from build123d import *

# Parameters (mm, degrees)
F0_R        = 1.15
F1_DEPTH    = 4
F2_R        = 1.5
F3_DEPTH    = 5
F4_T1_DEPTH = 16
F5_R        = 0.49999


# Not quite as in the source:
# - a fillet or chamfer that OpenCascade refuses, or shapes differently, is made with other operations: its cross-section is extruded or revolved along the edge and cut away or added
# - a fillet or chamfer is up to 0.001 mm smaller than in the source, because OpenCascade refuses the exact size


with BuildPart() as f1:
    # F0 (on Front) → F1 (new body)
    with BuildSketch(Plane.XZ):
        with BuildLine():
            Line((-3.5, -3.1), (5, -3.1))
            Line((5, -3.1), (5, 3.1))
            Line((5, 3.1), (-3.5, 3.1))
            ThreePointArc((-3.5, 3.1), (-3.9393398282, 2.0393398282), (-5, 1.6))
            Line((-5, 1.6), (-5, -1.6))
            ThreePointArc((-5, -1.6), (-3.9393398282, -2.0393398282), (-3.5, -3.1))
        make_face()
        with Locations((2.7, 0)):
            Circle(F0_R, mode=Mode.SUBTRACT)
    extrude(amount=F1_DEPTH)

    # F2 (on face) → F3 (cut)
    with BuildSketch(Plane(origin=(-5, 0, 0), x_dir=(0, -1, 0), z_dir=(-1, 0, 0))):
        with Locations((2, 0)):
            Circle(F2_R)
    extrude(amount=-F3_DEPTH, mode=Mode.SUBTRACT)

    # F4: fillet of radius 1.5 on 4 edges, made by hand

    # F4_s2 → F4_t1 (cut)
    with BuildSketch(Plane.YZ.offset(-7.25)):
        with BuildLine():
            ThreePointArc((0, 1.6), (-0.4393398282, 2.6606601718), (-1.5, 3.1))
            Line((-1.5, 3.1), (0, 3.1))
            Line((0, 3.1), (0, 1.6))
        make_face()
        with BuildLine():
            ThreePointArc((-4, 1.6), (-3.5606601718, 2.6606601718), (-2.5, 3.1))
            Line((-2.5, 3.1), (-4, 3.1))
            Line((-4, 3.1), (-4, 1.6))
        make_face()
        with BuildLine():
            ThreePointArc((-2.5, -3.1), (-3.5606601718, -2.6606601718), (-4, -1.6))
            Line((-4, -1.6), (-4, -3.1))
            Line((-4, -3.1), (-2.5, -3.1))
        make_face()
        with BuildLine():
            ThreePointArc((-1.5, -3.1), (-0.4393398282, -2.6606601718), (0, -1.6))
            Line((0, -1.6), (0, -3.1))
            Line((0, -3.1), (-1.5, -3.1))
        make_face()
    extrude(amount=F4_T1_DEPTH, mode=Mode.SUBTRACT)

    # F5 (radius 0.5 in the source; OpenCascade refuses exactly that, so slightly less here)
    f5_edges = [f1.edges().sort_by_distance(p)[0] for p in [
        (-5, 0, 0),
        (-5, -4, 0),
    ]]
    fillet(f5_edges, radius=F5_R)


solid = f1.part
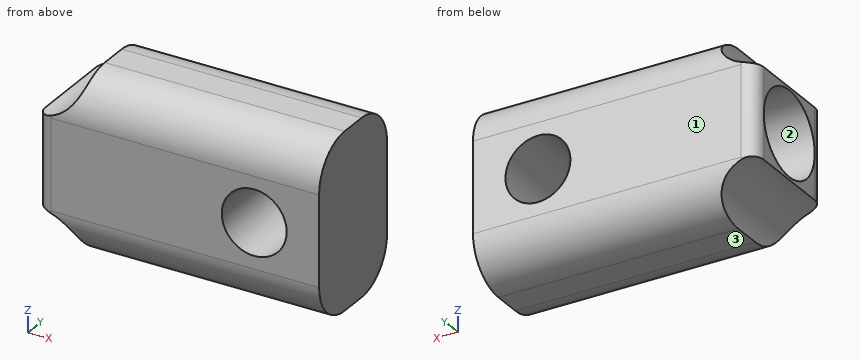
The listing builds one solid part. Answer for the finished solid, in the listing's coordinates (mm). Face numbers are marked on the shaded views. Round coordinates to 2 decimals unless told otherwise and drop trailing zeros. Order: outer loops, then holes, each group sorted by start corner. A loop starts at its lowest first (then second) coordinate and runs counter-clockwise, first axis right, second up. Notation, with made-up numbers: (65.5, 74.5) - (96.5, 74.5) arc R10 cw to (96.5, 78.5) - close; hole circle Ø6 at (38.25, 45.25). An arc over 180 degrees is marked (long way). Write item = value, one per line. Start each with the question number.
1) Given pin 1 (1.8 mm diameter, centred on x = 2.7, z = 0, fed in from +Y), flat-ended and moving along its own axis, determine where the tip first touches the part or whether it passes through.
2) Section D-D, the plane x = 0.25 is taken. Write down the section's boundary in (y, z).
3) Section B-B, the plane x = 2.7 is taken. Write down the section's boundary in (y, z), plus the area to 3 significant figures.
4) Section C-C, the plane y = -2 is taken. Write down the section's boundary in (x, z), plus the area to 3 significant figures.
5) For a pull along Y with two mould halves and no side action, classify the marked faces 1, 2 and 3 as released by +Y, released by -Y, zero draft, split by the parting line, or undercut.
6) Straight lines are drawn through the part: L1, parallel to Z at x = 2.7, y = -2; L2, parallel to X at y = -2.3, z = 0.5; L3, parallel to X at y = -2.1, z = 1. For each, find the intervals that lie inside material, in ascending order.
Results list:
q1.pin_1 = through
q2.outline = (-4, -1.6) arc R1.5 ccw to (-2.5, -3.1) - (-1.5, -3.1) arc R1.5 ccw to (0, -1.6) - (0, 1.6) arc R1.5 ccw to (-1.5, 3.1) - (-2.5, 3.1) arc R1.5 ccw to (-4, 1.6) - close
q3.outline = (-4, -1.6) arc R1.5 ccw to (-2.5, -3.1) - (-1.5, -3.1) arc R1.5 ccw to (0, -1.6) - (0, -1.15) - (-4, -1.15) - close; (-4, 1.15) - (0, 1.15) - (0, 1.6) arc R1.5 ccw to (-1.5, 3.1) - (-2.5, 3.1) arc R1.5 ccw to (-4, 1.6) - close
q3.area = 13.7 mm^2
q4.outline = (-5, -1.6) arc R1.5 cw to (-3.5, -3.1) - (5, -3.1) - (5, 3.1) - (-3.5, 3.1) arc R1.5 cw to (-5, 1.6) - (-5, 1.5) - (0, 1.5) - (0, -1.5) - (-5, -1.5) - close; hole circle Ø2.3 at (2.7, 0)
q4.area = 39.3 mm^2
q5.face_1 = released by +Y
q5.face_2 = undercut
q5.face_3 = zero draft
q6.L1 = -3.1 to -1.15, 1.15 to 3.1
q6.L2 = 0 to 1.66, 3.74 to 5
q6.L3 = 0 to 2.13, 3.27 to 5
